Geometry check sheet. Reference: the model listing, model coordinates, mm. Give positions to 0.01 mm unless a question says otherwise; leave off trailing zeros. Order: outer loops, then holes, each group sorted by start corner. A loop starts at its lowest first (then second) coordinate and runs counter-clockwise, first axis right, second up. Notation, with made-up numbers: M 36.25,4 L 82.25,4 A23 ccw 82.25,20 Z; hole C 81.25,-25 d9. An arc over 180 degrees is marked long. Answer as CSV lines item,"result". Start each with the question number.
Q1. Mould release check, pull along Y, two halves, no side actions. Record for faces 1 (the flat face through (0, -25, 25)), 2 (the flat face through (25, -50, 25)), 3 (the flat face through (25, 0, 25)), 4 (the cylindrical face through (24.65, -28.05, 13.74)): +Y half, -Y half, draft (parallel to the pull), parting line (faces both ways), or undercut.
Q2. Section check B-B, the plane z = 15. Record the boundary of the cut face in (x, y).
Q3. Thickness scan on line 1 (Z direction, x = 16, y = -25). Record the ranges inside material, lowest first.
Q4. Go/stop test with a flat-tipped pin: pin 1 (4 mm diameter, centred on y = -25, z = 15, fed in from -X). Record where the tip stops, or that it passes through.
Q5. Section check A-A, the plane y = -25. Record the boundary of the cut face in (x, z), then the cut area to 3 significant figures.
```python
from build123d import *

# Parameters (mm, degrees)
F0_W     = 50
F0_H     = 50
F1_DEPTH = 50
F3_D     = 6.6


with BuildPart() as f1:
    # F0 (on Front) → F1 (new body)
    with BuildSketch(Plane.XZ):
        with Locations((25, 25)):
            Rectangle(F0_W, F0_H)
    extrude(amount=F1_DEPTH)

    # F3 (through all)
    with Locations(Plane.YZ.offset(50)):
        with Locations((-25, 15)):
            Hole(F3_D / 2)


solid = f1.part
```
Answer block:
1,face 1,"draft"
1,face 2,"-Y half"
1,face 3,"+Y half"
1,face 4,"undercut"
2,outline,"M 0,-50 L 50,-50 L 50,-28.3 L 0,-28.3 Z; M 0,-21.7 L 50,-21.7 L 50,0 L 0,0 Z"
3,line 1,"z = 0 to 11.7, 18.3 to 50"
4,pin 1,"passes through"
5,outline,"M 0,0 L 50,0 L 50,11.7 L 0,11.7 Z; M 0,18.3 L 50,18.3 L 50,50 L 0,50 Z"
5,area,"2,170 mm2"
